The model under review builds one solid part; all positions refer to its coordinate system, in mm. Face numbers are marked on the shaded views. Round coordinates to 2 decimals unless told otherwise and drop trailing zeros. Order: outer loops, then holes, each group sorted by start corner. A loop starts at its lowest first (then second) coordinate and runs counter-clockwise, first axis right, second up. Notation, with made-up numbers: M 52.5,72.5 L 99.5,72.5 A31 cw 99.5,110.5 Z; hole C -27.75,-32.75 d3. An arc over 180 degrees is marked long. Answer as a JSON object with one key per item and string values. Group by question number.
1) Consider section C-C, the plane y = 8. Write out the cut boundary in (x, z).
2) Consider section B-B, the plane z = 0. Write out the cut boundary in (x, y), then the cut area to 3 significant figures.
3) To check wall thickness, follow line 1 (X direction, y = 12, z = 0); line 2 (Y direction, x = 14.5, z = -20.5); line 3 (Z direction, x = -1.5, y = 29.5). State the ranges of each line that lie inside material, in increasing order.
4) Consider section A-A, the plane x = 0. Write out the cut boundary in (y, z).
5) Insertion check: pin 1 Ø4 at (x, z) = (13.5, 13.5) entering from +Y; pin 2 Ø1.5 at (y, z) = (8, 19.5) entering from +X. Each pin has a flat end and moves straight along its axis. Give the tip position at first contact, or say it passes through.
6) Consider section D-D, the plane x = 12. Write out the cut boundary in (y, z).
7) The part is to be moulded in two halves that separate along Z. For the marked faces 1, 2 and 3, say which applies: +Z half, -Z half, draft (parallel to the pull), parting line (faces both ways), or undercut.
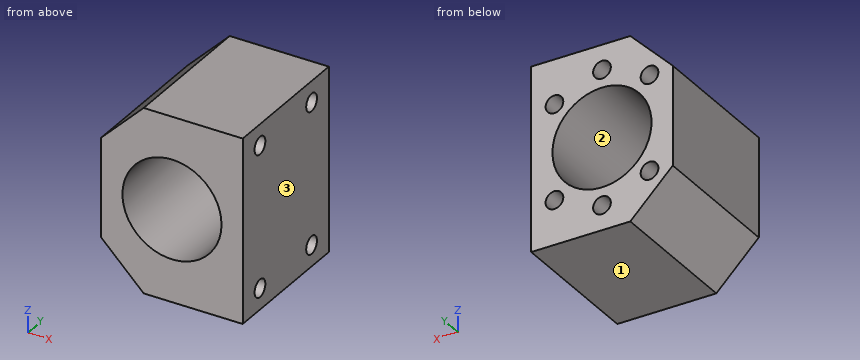
```python
from build123d import *

# Parameters (mm, degrees)
SKETCH_1_R          = 14
EXTRUDE_1_DEPTH     = 40
SKETCH_2_R          = 2.5
CUT_EXTRUDE_1_DEPTH = 10
SKETCH_3_R          = 2.5
CUT_EXTRUDE_2_DEPTH = 10


with BuildPart() as part:
    # Эскиз1 → Бобышка-Вытянуть1 (new body)
    with BuildSketch(Plane(origin=(0, 0, 0), x_dir=(1, 0, 0), z_dir=(0, 1, 0))):
        Polygon((-20, 14), (-8, 26), (20, 26), (20, -26), (-8, -26), (-20, -14), align=None)
        Circle(SKETCH_1_R, mode=Mode.SUBTRACT)
    extrude(amount=EXTRUDE_1_DEPTH)

    # Эскиз2 → Вырез-Вытянуть1 (cut)
    with BuildSketch(Plane(origin=(0, 40, 0), x_dir=(1, 0, 0), z_dir=(0, 1, 0))):
        with Locations((0, 19)):
            Circle(SKETCH_2_R)
        with Locations((13.435028843, 13.435028843)):
            Circle(SKETCH_2_R)
        with Locations((13.435028843, -13.435028843)):
            Circle(SKETCH_2_R)
        with Locations((0, -19)):
            Circle(SKETCH_2_R)
        with Locations((-13.435028843, -13.435028843)):
            Circle(SKETCH_2_R)
        with Locations((-13.435028843, 13.435028843)):
            Circle(SKETCH_2_R)
    extrude(amount=-CUT_EXTRUDE_1_DEPTH, mode=Mode.SUBTRACT)

    # Эскиз3 → Вырез-Вытянуть2 (cut)
    with BuildSketch(Plane(origin=(20, 0, 0), x_dir=(0, 0, -1), z_dir=(1, 0, 0))):
        with Locations((-20, 32)):
            Circle(SKETCH_3_R)
        with Locations((20, 32)):
            Circle(SKETCH_3_R)
        with Locations((20, 8)):
            Circle(SKETCH_3_R)
        with Locations((-20, 8)):
            Circle(SKETCH_3_R)
    extrude(amount=-CUT_EXTRUDE_2_DEPTH, mode=Mode.SUBTRACT)


solid = part.part
```
Results list:
{
 "1": {"outline": "M -20,-14 L -8,-26 L 20,-26 L 20,-22.5 L 10,-22.5 L 10,-17.5 L 20,-17.5 L 20,17.5 L 10,17.5 L 10,22.5 L 20,22.5 L 20,26 L -8,26 L -20,14 Z; hole C 0,0 d28"},
 "2": {"outline": "M -20,0 L -14,0 L -14,40 L -20,40 Z; M 14,0 L 20,0 L 20,40 L 14,40 Z", "area": "480 mm^2"},
 "3": {"line 1": "-20 to -14, 14 to 20", "line 2": "0 to 5.55, 10.45 to 29.55, 34.45 to 40", "line 3": "-26 to -13.92, 13.92 to 26"},
 "4": {"outline": "M 0,-26 L 40,-26 L 40,-21.5 L 30,-21.5 L 30,-16.5 L 40,-16.5 L 40,-14 L 0,-14 Z; M 0,14 L 40,14 L 40,16.5 L 30,16.5 L 30,21.5 L 40,21.5 L 40,26 L 0,26 Z"},
 "5": {"pin 1": "y = 30", "pin 2": "x = 10"},
 "6": {"outline": "M 0,-26 L 40,-26 L 40,-15.48 L 30,-15.48 L 30,-11.39 L 40,-11.39 L 40,-7.21 L 0,-7.21 Z; M 0,7.21 L 40,7.21 L 40,11.39 L 30,11.39 L 30,15.48 L 40,15.48 L 40,26 L 0,26 Z; hole C 8,-20 d5; hole C 8,20 d5; hole C 32,-20 d5; hole C 32,20 d5"},
 "7": {"face 1": "-Z half", "face 2": "undercut", "face 3": "draft"}
}
